Design review of the part built by this model. Coordinates are the model's own, in mm. A direction names the side the tool comes from. Round coordinates to 2 decimals unless told otherwise and drop trailing zeros. Write each loop counter-clockwise with the first axis right and the second up, starting at its lowest first coordinate (ties: lowest second). Pieces come first, ordered by that corner, then holes. Notation, with made-up numbers: (77.25, -8) -> (133.25, -8) arc R34 cw to (133.25, 29) -> close; hole circle Ø10 at (-28.5, 87). An arc over 180 degrees is marked (long way). Write item = value, one per line. Start each with the question number.
Item 1: Add section B-B, the plane y = 5.75. State the section outline as (x, z) points (3 decimals), then the cut area to 3 significant figures.
Item 2: Add section C-C, the plane x = -25. State the section outline as (y, z) points (3 decimals).
Item 3: Add section A-A, the plane z = 1.75. State the section outline as (x, y) points, then the cut area to 3 significant figures.
Item 4: Machinability: for faces 1 (the flat face through (0, 11.36, 0)), 2 (the flat face through (1, 6, 7.525)), 3 (the cylindrical face through (37, -1, -8)), which of the approach directions +Z, -Z, +X, -X, +Y, -Y give a long, thin tool a straight path to every point of the face, cutting with its end or side? Answer none if there is none.
Item 5: To check wall thickness, follow L1, parallel to Z at x = -15.5, y = 0.5 (3 decimals); L2, parallel to Z at x = -15, y = 10 (3 decimals); L3, parallel to Y at x = 4, z = 5. State the ranges of each line that lie inside material, in increasing order.
Item 6: For pin 1 Ø1.5 at (x, y) = (5.5, 1.5) entering from +Z (3 decimals); pin 2 Ø3 at (x, y) = (-5, 5) entering from -Z (3 decimals); pin 3 Ø1.5 at (y, z) = (8.5, 4.5) entering from -X; pin 4 Ø4 at (x, z) = (-21, -3.5) entering from -Y, all flat-tipped, find the tip position at first contact; note any pin that passes through.
Item 7: Mouldability with a two-part tool opening along X and no side actions: class faces 4 (the flat face through (0, 1.2, -8)), 5 (the flat face through (-38.1, 1, 0)), 6 (the flat face through (0, 0, -9)) as released by +X, released by -X, zero draft, split by the parting line, or undercut.
from build123d import *

# Parameters (mm, degrees)
SKETCH1_W               = 76.2
SKETCH1_H               = 19.05
BOSS_EXTRUDE1_DEPTH     = 1.2
BOSS_EXTRUDE2_START     = -2
BOSS_EXTRUDE2_DEPTH     = 15.05
SHELL1_START            = -6.325
SHELL1_DEPTH            = 12.65
SKETCH3_R               = 0.6
BOSS_EXTRUDE3_DEPTH     = 1.2
MIRROR2_COPY_1_SKETCH_R = 0.6
MIRROR2_COPY_1_DEPTH    = 1.2


# Read off the part's stored shape, not the designer's step: Shell1
with BuildPart() as part:
    # Sketch1 → Boss-Extrude1 (new body)
    with BuildSketch(Plane(origin=(0, 0, 0), x_dir=(1, 0, 0), z_dir=(0, 1, 0))):
        Rectangle(SKETCH1_W, SKETCH1_H)
    extrude(amount=BOSS_EXTRUDE1_DEPTH)

    # Sketch2 → Boss-Extrude2 (add)
    with BuildSketch(Plane.XY.offset(9.525).offset(BOSS_EXTRUDE2_START)):
        Polygon((-36.9, 1.2), (-26.74, 11.36), (26.74, 11.36), (36.9, 1.2), align=None)
    extrude(amount=-BOSS_EXTRUDE2_DEPTH)

    # Shell1 outline → Shell1 (cut)
    with BuildSketch(Plane.XY.offset(SHELL1_START)):
        Polygon((26.242943725, 10.16), (-26.242943725, 10.16), (-36.402943725, 0), (36.402943725, 0), align=None)
    extrude(amount=SHELL1_DEPTH, mode=Mode.SUBTRACT)

    # Sketch3 → Boss-Extrude3 (add)
    with BuildSketch(Plane.XZ):
        with Locations(Location((-36.402943725, 7.924066334, 0), (0, 0, 90))):
            Circle(SKETCH3_R)
    boss_extrude3 = extrude(amount=BOSS_EXTRUDE3_DEPTH)

    # Mirror1: Boss-Extrude3 across plane
    add(boss_extrude3.mirror(Plane.XY))

    # Mirror2: Boss-Extrude3 across plane
    add(boss_extrude3.mirror(Plane(origin=(0, 0, 0), x_dir=(0, 0, 1), z_dir=(1, 0, 0))))

    # Mirror2 copy 1 sketch → Mirror2 copy 1 (add)
    with BuildSketch(Plane(origin=(0, 0, 0), x_dir=(-1, 0, 0), z_dir=(0, -1, 0))):
        with Locations(Location((-36.402943725, 7.924066334, 0), (0, 0, 90))):
            Circle(MIRROR2_COPY_1_SKETCH_R)
    extrude(amount=MIRROR2_COPY_1_DEPTH)


solid = part.part
Result set:
q1.outline = (-32.35, -7.525) -> (32.35, -7.525) -> (32.35, 7.525) -> (-32.35, 7.525) -> close; hole (-30.653, -6.325) -> (30.653, -6.325) -> (30.653, 6.325) -> (-30.653, 6.325) -> close
q1.area = 198 mm²
q2.outline = (0, -9.525) -> (1.2, -9.525) -> (1.2, -7.525) -> (11.36, -7.525) -> (11.36, 7.525) -> (1.2, 7.525) -> (1.2, 9.525) -> (0, 9.525) -> (0, 6.325) -> (10.16, 6.325) -> (10.16, -6.325) -> (0, -6.325) -> close
q3.outline = (-38.1, 0) -> (-36.4, 0) -> (-26.24, 10.16) -> (26.24, 10.16) -> (36.4, 0) -> (38.1, 0) -> (38.1, 1.2) -> (36.9, 1.2) -> (26.74, 11.36) -> (-26.74, 11.36) -> (-36.9, 1.2) -> (-38.1, 1.2) -> close
q3.area = 102 mm²
q4.face_1 = +Z, -Z, +X, -X, +Y
q4.face_2 = +Z, +X, -X, +Y
q4.face_3 = -Y
q5.L1 = -9.525 to -6.325, 6.325 to 9.525
q5.L2 = -7.525 to -6.325, 6.325 to 7.525
q5.L3 = 10.16 to 11.36
q6.pin_1 = 9.525
q6.pin_2 = -7.525
q6.pin_3 = -30.35
q6.pin_4 = 10.16
q7.face_4 = zero draft
q7.face_5 = released by -X
q7.face_6 = undercut
